Source: CAD feature listing. Evaluate the final solid. Frame: model axes, mm. Coordinates: 2 decimals unless noted, no trailing zeros. Write each loop counter-clockwise with the first axis right and the second up, starting at its lowest first coordinate (ties: lowest second). Pieces come first, ordered by that corner, then holes. Notation, with made-up numbers: M 67,7 L 122,7 A15 cw 122,27 Z; hole C 0,15 d8. An arc over 180 degrees is marked long. One line per item, written item: value. Start each with the question number.
Item 1: Cut plane A-A, the plane x = 12.7. Output: boundary loops of the cut face in (y, z) (3 decimals), then the cut area to 3 significant figures.
Item 2: Cut plane C-C, the plane y = 87.5. Output: boundary loops of the cut face in (x, z) (3 decimals), then the cut area to 3 significant figures.
Item 3: Cut plane D-D, the plane z = -1.45. State how many separate pieces and enclosed holes the cut face has, then the cut area to 3 significant figures.
Item 4: Mould query, pull axis Y, two halves, no side actions, for faces 1 (the flat face through (0, 77, -2)), 2 (the flat face through (52, 152.4, -2)), 3 (the flat face through (50, 0, -2)), 4 (the cylindrical face through (77.075, 43.105, -1.61)). Classes: released by +Y, released by -Y, zero draft, split by the parting line, or undercut.
Item 5: Cut plane B-B, the plane x = 50.8. Output: boundary loops of the cut face in (y, z) (1 decimal).
Item 6: Ray query, L1, parallel to X at y = 44.45, z = -0.7; L2, parallel to Y at x = 50.8, z = -1.15; L3, parallel to X at y = 12.7, z = -0.85 (3 decimals). Return the intervals inside material, ascending. Write a range as from..to.
Item 7: Pin query (flat end, axial travel): P1, Ø20.5, axis at x = 50.8, y = 93.66, coming from the +Z side. Return the tip coordinate at first contact, or that it passes through.
Autodesk Inventor part; units mm, degrees
ref_plane "YZ Plane" through (0, 0, 0) normal (1, 0, 0) x (0, 1, 0)
ref_plane "XZ Plane" through (0, 0, 0) normal (0, 1, 0) x (-1, 0, 0)
ref_plane "XY Plane" through (0, 0, 0) normal (0, 0, 1) x (1, 0, 0)
sketch "Sketch1" plane through (0, 0, 0) normal (0, 0, 1) x (1, 0, 0)
  line L0 (0, 0) -> (101.6, 0)
  line L1 (101.6, 0) -> (101.6, 152.4)
  line L2 (101.6, 152.4) -> (0, 152.4)
  line L3 (0, 152.4) -> (0, 0)
  point P0 (22.4155, 44.45)
  point P1 (79.1845, 44.45)
  point P2 (50.8, 141.9352)
  point P3 (50.8, 93.6625)
  point P4 (12.7, 12.7)
  point P5 (88.9, 12.7)
  dimension "d0" = 152.4
  dimension "d1" = 101.6
  dimension "d2" = 44.45
  dimension "d3" = 49.2125
  dimension "d4" = 97.4852
  dimension "d5" = 56.769
  dimension "d6" = 28.3845
  dimension "d7" = 12.7
  dimension "d8" = 12.7
  dimension "d9" = 12.7
  dimension "d10" = 50.8
extrude "Extrusion1" add sketch "Sketch1" against normal blind 3.175
hole "Hole1" at (22.4155, 44.45, 0) at (79.1845, 44.45, 0) at (50.8, 141.9352, 0) direction (0, 0, -1) diameter 5.0038 depth 25.4 tip angle 118
hole "Hole2" at (12.7, 12.7, 0) at (88.9, 12.7, 0) direction (0, 0, -1) diameter 6.35 depth 25.4 tip angle 118
hole "Hole3" at (50.8, 93.6625, 0) direction (0, 0, -1) diameter 25.4 depth 25.4 tip angle 118
properties part number "window motor plate"
From the geometry:
1. outline: M 0,-3.175 L 9.525,-3.175 L 9.525,0 L 0,0 Z; M 15.875,-3.175 L 152.4,-3.175 L 152.4,0 L 15.875,0 Z
1. area: 464 mm²
2. outline: M 0,-3.175 L 39.695,-3.175 L 39.695,0 L 0,0 Z; M 61.905,-3.175 L 101.6,-3.175 L 101.6,0 L 61.905,0 Z
2. area: 252 mm²
3. separate pieces: 1
3. enclosed holes: 6
3. area: 14,900 mm²
4. face 1: zero draft
4. face 2: released by +Y
4. face 3: released by -Y
4. face 4: undercut
5. outline: M 0,-3.2 L 81,-3.2 L 81,0 L 0,0 Z; M 106.4,-3.2 L 139.4,-3.2 L 139.4,0 L 106.4,0 Z; M 144.4,-3.2 L 152.4,-3.2 L 152.4,0 L 144.4,0 Z
6. L1: x = 0..19.91, 24.92..76.68, 81.69..101.6
6. L2: y = 0..80.96, 106.36..139.43, 144.44..152.4
6. L3: x = 0..9.525, 15.875..85.725, 92.075..101.6
7. P1: passes through
